from build123d import *

# Parameters (mm, degrees)
RESSALTO_EXTRUS_O1_DEPTH       = 12
FURO_COM_FOLGA_DE_M51_D        = 5.5
ESBO_O9_R                      = 7
CORTE_EXTRUS_O3_DEPTH          = 5
CORTE_EXTRUS_O4_DEPTH          = 5.26
FURO_DE_DI_METRO_4_0_4_1_D     = 4
FURO_DE_DI_METRO_4_0_4_1_DEPTH = 6.74
FURO_DE_DI_METRO_4_0_4_1_TIP   = 1.201721238


with BuildPart() as part:
    # Esboço1 → Ressalto-extrusão1 (new body)
    with BuildSketch(Plane.XY):
        Polygon((69.044771166, -26.921923077), (81.044771166, -38.921923077), (81.044771166, -66.921923077), (51.044771166, -66.921923077), (51.044771166, -38.921923077), (63.044771166, -26.921923077), align=None)
    extrude(amount=RESSALTO_EXTRUS_O1_DEPTH)

    # Furo com folga de M51 (through all)
    with Locations(Plane.XY.offset(12)):
        with Locations((66.044771166, -53.121923077)):
            Hole(FURO_COM_FOLGA_DE_M51_D / 2)

    # Esboço9 → Corte-extrusão3 (cut)
    with BuildSketch(Plane.XY.offset(12)):
        with Locations((66.044771166, -53.121923077)):
            Circle(ESBO_O9_R)
    extrude(amount=-CORTE_EXTRUS_O3_DEPTH, mode=Mode.SUBTRACT)

    # Esboço10 → Corte-extrusão4 (cut)
    with BuildSketch(Plane.XY.offset(12)):
        Polygon((51.044771166, -41.251110711), (51.044771166, -38.921923077), (63.044771166, -26.921923077), (69.044771166, -26.921923077), (81.044771166, -38.921923077), (81.044771166, -41.251110711), align=None)
    extrude(amount=-CORTE_EXTRUS_O4_DEPTH, mode=Mode.SUBTRACT)

    # Furo de diâmetro Ø4.0 (4)1
    with Locations(Plane.XY.offset(6.74)):
        with Locations((66.044771166, -37.251110711)):
            Hole(FURO_DE_DI_METRO_4_0_4_1_D / 2, depth=FURO_DE_DI_METRO_4_0_4_1_DEPTH)
            with Locations((0, 0, -(FURO_DE_DI_METRO_4_0_4_1_DEPTH + FURO_DE_DI_METRO_4_0_4_1_TIP / 2))):  # 118° drill point
                Cone(0, FURO_DE_DI_METRO_4_0_4_1_D / 2, FURO_DE_DI_METRO_4_0_4_1_TIP, mode=Mode.SUBTRACT)


solid = part.part
The listing builds one solid part. Answer for the finished solid, in the listing's coordinates (mm). A direction names the side the tool comes from. Coordinates: 2 decimals unless noted, no trailing zeros. Loops run counter-clockwise (first coordinate to the right, second up) from the corner with the lowest first, then second, coordinate; pieces in that order, holes last. Notation, with made-up numbers: M -16,75 L -3,75 A28 cw -3,94 Z; hole C 81.5,82.25 d2. An arc over 180 degrees is marked long. Answer in a Markdown table with one row per item.
1) Find section A-A (x = 64.5). Determine the outline of the cut face in (y, z), then the cut area to 3 significant figures.
Answers below:
| item | result |
|---|---|
| outline | M -66.92,0 L -55.4,0 L -55.4,7 L -59.95,7 L -59.95,12 L -66.92,12 Z; M -50.85,0 L -38.52,0 L -38.52,6.74 L -41.25,6.74 L -41.25,12 L -46.29,12 L -46.29,7 L -50.85,7 Z; M -35.98,0 L -26.92,0 L -26.92,6.74 L -35.98,6.74 Z |
| area | 287 mm^2 |
2) Determine the mould class of faces 4 (the flat face through (66, -34, 6.74)), 5 (the flat face through (56.961, -33.006, 3.323)), 6 (the cylindrical face through (66.641, -55.807, 3.451)), 7 (the cylindrical face through (60.49, -57.38, 9.54)) for opening direction Y: released by +Y, released by -Y, zero draft, split by the parting line, or undercut.
Answers below:
| item | result |
|---|---|
| face 4 | zero draft |
| face 5 | released by +Y |
| face 6 | undercut |
| face 7 | undercut |
3) Which of the six approach directions +Z, -Z, +X, -X, +Y, -Y give full straight-line access (tool end or side, diameter ignored) to faces 1 (the flat face through (74.961, -32.838, 3.323)), 2 (the flat face through (65.9, -56.1, 7)), 3 (the flat face through (66, -41.251, 9))?
Answers below:
| item | result |
|---|---|
| face 1 | +Z, -Z, +X, +Y |
| face 2 | +Z |
| face 3 | +Z, +X, -X, +Y |
4) Given pin 1 (2 mm diameter, centred on x = 72, z = 8.5, fed in from +Y); pin 2 (6.5 mm diameter, centred on x = 66.04, y = -53.12, fed in from +Z); pin 3 (4.5 mm diameter, centred on x = 68, y = -32, fed in from +Z), each flat-ended and moving along its own axis, determine where each tip first touches the part or whether it passes through.
Answers below:
| item | result |
|---|---|
| pin 1 | y = -41.25 |
| pin 2 | z = 7 |
| pin 3 | z = 6.74 |
5) Find the intervals of material crossed by probe 1 along X at (y, z) = (-53, 6.5); probe 2 along Z at (x, y) = (73, -33.5); probe 3 along Y at (x, z) = (72.5, 10), in increasing order.
Answers below:
| item | result |
|---|---|
| probe 1 | 51.04 to 63.3, 68.79 to 81.04 |
| probe 2 | 0 to 6.74 |
| probe 3 | -66.92 to -55.83, -50.41 to -41.25 |
6) Find section C-C (z = 11.25). Determine the outline of the cut face in (x, y).
Answers below:
| item | result |
|---|---|
| outline | M 51.04,-66.92 L 81.04,-66.92 L 81.04,-41.25 L 51.04,-41.25 Z; hole C 66.04,-53.12 d14 |
7) Find section D-D (z = 5.75). Determine the outline of the cut face in (x, y), then the cut area to 3 significant figures.
Answers below:
| item | result |
|---|---|
| outline | M 51.04,-66.92 L 81.04,-66.92 L 81.04,-38.92 L 69.04,-26.92 L 63.04,-26.92 L 51.04,-38.92 Z; hole C 66.04,-53.12 d5.5; hole C 66.04,-37.25 d4 |
| area | 1,020 mm^2 |
8) Find section B-B (y = -52). Determine the outline of the cut face in (x, z), then the cut area to 3 significant figures.
Answers below:
| item | result |
|---|---|
| outline | M 51.04,0 L 63.53,0 L 63.53,7 L 59.14,7 L 59.14,12 L 51.04,12 Z; M 68.56,0 L 81.04,0 L 81.04,12 L 72.95,12 L 72.95,7 L 68.56,7 Z |
| area | 256 mm^2 |
